Can you work these out from the model? Positions are in its coordinate system, mm. Coordinates: 2 decimals unless noted, no trailing zeros. Write each loop counter-clockwise with the first axis right and the second up, starting at its lowest first coordinate (ties: lowest second). Pieces come first, ordered by that corner, then holes. Notation, with made-up numbers: (23, -12.75) - (31, -12.75) arc R23 cw to (31, 16.25) - close; hole circle Ø6 at (27.5, -14.75). An arc over 180 degrees is marked (long way). Use one line per item in the form item = value. Start each with the question number.
(1) Thinking about a two-plate mould opening in Z: for faces 1 (the face through (0.24, 236.47, 30.94)), 2 (the face through (0, 0, 31)), 3 (the face through (-0.25, 125.24, 46.99)), which applies, pulls with the +Z half, pulls with the -Z half, needs draft (parallel to the pull), parting line crosses it, or undercut?
(2) If I drill on probe 1 along Y at (x, z) = (-15, 35); probe 2 along Y at (x, z) = (-13.5, 35.5); probe 3 along Z at (x, y) = (0, 142), over which ranges is the centre line in solid material (lowest first)? Write a range as from..to.
(3) For pin 1 Ø5 at (x, y) = (-13.5, 134.5) entering from +Z; pin 2 Ø5 at (x, y) = (13.5, 124) entering from -Z; pin 3 Ø4 at (x, y) = (9, 82.5) entering from -Z, each with a flat end and sliding along its axis, tell me the tip position at first contact or that it passes through.
(4) If we section it at B-B on z = 27: Give the number of separate pieces and of enclosed holes in the cut face, then the cut area to 3 significant figures.
(5) If we section it at A-A on y = 228.6: Please give me the cut outline in (x, z).
```python
from build123d import *

# Parameters (mm, degrees)
BOSS_EXTRUDE1_DEPTH = 254
SKETCH2_R           = 7.9375
CUT_EXTRUDE1_DEPTH  = 261.833544861
FILLET1_R           = 1.27


with BuildPart() as part:
    # Sketch1 → Boss-Extrude1 (new body)
    with BuildSketch(Plane(origin=(0, 0, 0), x_dir=(1, 0, 0), z_dir=(0, 1, 0))):
        with BuildLine():
            Line((-18.0975, -16.448172274), (-18.0975, -43.365200262))
            ThreePointArc((-18.0975, -43.365200262), (0, -46.99), (18.0975, -43.365200262))
            Line((18.0975, -43.365200262), (18.0975, -16.448172274))
            ThreePointArc((18.0975, -16.448172274), (0, -18.628441839), (-18.0975, -16.448172274))
        make_face()
    extrude(amount=BOSS_EXTRUDE1_DEPTH)

    # Sketch2 → Cut-Extrude1 (cut, through all)
    with BuildSketch(Plane(origin=(18.0975, 0, 0), x_dir=(0, 0, -1), z_dir=(1, 0, 0))):
        with Locations((-29.906686268, 228.6)):
            Circle(SKETCH2_R)
        with Locations((-29.906686268, 25.4)):
            Circle(SKETCH2_R)
    extrude(amount=-CUT_EXTRUDE1_DEPTH, mode=Mode.SUBTRACT)

    # Fillet1
    fillet1_edges = [part.edges().sort_by_distance(p)[0] for p in [
        (0, 254, 46.99),
        (18.0975, 254, 29.906686268),
        (-18.0975, 228.6, 37.844186268),
        (18.0975, 228.6, 37.844186268),
        (-18.0975, 25.4, 37.844186268),
        (18.0975, 25.4, 37.844186268),
        (18.0975, 0, 29.906686268),
        (0, 0, 46.99),
        (-18.0975, 0, 29.906686268),
        (18.0975, 127, 43.365200262),
        (-18.0975, 127, 43.365200262),
        (-18.0975, 127, 16.448172274),
        (-18.0975, 254, 29.906686268),
    ]]
    fillet(fillet1_edges, radius=FILLET1_R)


solid = part.part
```
Reported:
q1.face_1 = undercut
q1.face_2 = needs draft
q1.face_3 = pulls with the +Z half
q2.probe_1 = 0..19.31, 31.49..222.51, 234.69..254
q2.probe_2 = 0..19.77, 31.03..222.97, 234.23..254
q2.probe_3 = 18.63..46.99
q3.pin_1 = 45.68
q3.pin_2 = 16.93
q3.pin_3 = 17.83
q4.separate_pieces = 3
q4.enclosed_holes = 0
q4.area = 8,120 mm2
q5.outline = (-18.1, 18.05) arc R1.27 ccw to (-16.55, 16.81) arc R76.2 cw to (18.1, 16.45) - (18.1, 20.7) arc R1.27 ccw to (16.83, 21.97) - (-16.83, 21.97) arc R1.27 ccw to (-18.1, 20.7) - close; (-18.1, 39.11) arc R1.27 ccw to (-16.83, 37.84) - (16.83, 37.84) arc R1.27 ccw to (18.1, 39.11) - (18.1, 42.51) arc R1.27 ccw to (17.29, 43.69) arc R46.99 ccw to (-17.29, 43.69) arc R1.27 ccw to (-18.1, 42.51) - close
